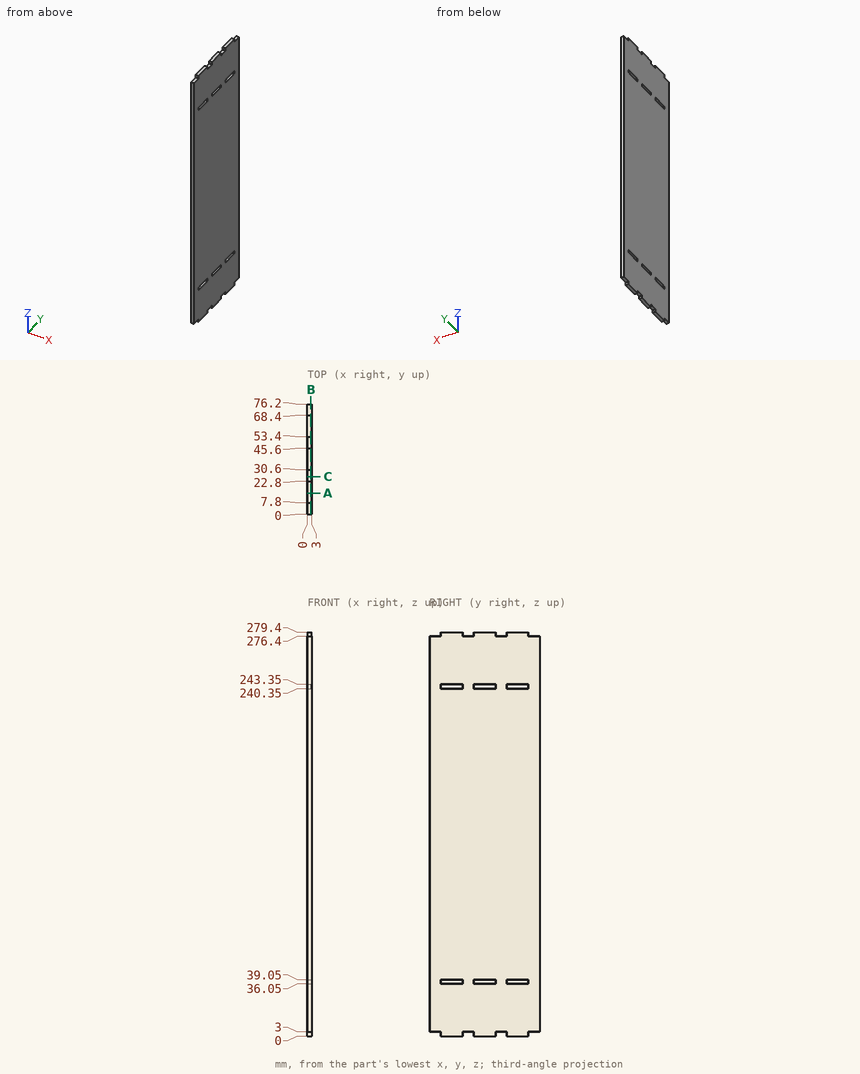
The figure shows three views and two pictorial views of one solid part (mm, origin at its lowest corner). Answer the questions. Give positions to 0.01 mm unless a question says otherwise; leave off trailing zeros. Loops run counter-clockwise (first coordinate to the right, second up) from the corner with the lowest first, then second, coordinate; pieces in that order, holes last. Notation, with made-up numbers: (77.25, 62) - (134.25, 62) arc R26 cw to (134.25, 80) - close; hole circle Ø4 at (-36.75, 58). An arc over 180 degrees is marked (long way). Use one line per item in the form item = value.
1. Section A-A on y = 14.5 is taken. Give the vertices of the cut face in (x, z), then the cut area to 3 significant figures.
Calculated:
outline = (0, 0) - (3, 0) - (3, 36.05) - (0, 36.05) - close; (0, 39.05) - (3, 39.05) - (3, 240.35) - (0, 240.35) - close; (0, 243.35) - (3, 243.35) - (3, 279.4) - (0, 279.4) - close
area = 820 mm^2
2. Section C-C on y = 26 is taken. Give the vertices of the cut face in (x, z), then the cut area to 3 significant figures.
Calculated:
outline = (0, 3) - (3, 3) - (3, 276.4) - (0, 276.4) - close
area = 820 mm^2
3. Find the intervals of material crossed by line 1 along Z through (x, y) = (1.5, 62.5); line 2 along Z through (x, y) = (0.9, 70), in increasing order. Write a range as [from, to].
Calculated:
line_1 = [0, 36.05], [39.05, 240.35], [243.35, 279.4]
line_2 = [3, 276.4]
4. Section B-B on x = 2.45 is taken. Count the separate pieces of the cut face and the enclosed holes in it, then the cut area to 3 significant figures.
Calculated:
separate_pieces = 1
enclosed_holes = 6
area = 20,800 mm^2
5. Given pin 1 Ø0.9 at (x, z) = (1.5, 1) entering from +Y; pin 2 Ø1.5 at (x, y) = (1, 26.5) entering from -Z; pin 3 Ø0.9 at (x, z) = (1, 277) entering from -Y, each flat-ended and moving along its own axis, determine where each tip first touches the part or whether it passes through.
Calculated:
pin_1 = 68.4
pin_2 = 3
pin_3 = 7.8
